Could you check a few things on this model? Use its own coordinates, in mm. Face numbers are marked on the shaded views. A direction names the side the tool comes from. Give positions to 0.01 mm unless a question says otherwise; leave off trailing zeros. Order: outer loops, then holes, each group sorted by start corner. A loop starts at its lowest first (then second) coordinate and runs counter-clockwise, first axis right, second up. Notation, with made-up numbers: (84, -30) -> (111, -30) arc R25 cw to (111, -13) -> close; hole circle Ø9 at (32.25, 10.5). An arc over 180 degrees is marked (long way). Write each question's results on one line, items separated by ' | '.
Autodesk Inventor part; units mm, degrees
ref_plane "YZ Plane" through (0, 0, 0) normal (1, 0, 0) x (0, 1, 0)
ref_plane "XZ Plane" through (0, 0, 0) normal (0, 1, 0) x (-1, 0, 0)
ref_plane "XY Plane" through (0, 0, 0) normal (0, 0, 1) x (1, 0, 0)
sketch "Schizzo1" plane through (0, 0, 0) normal (0, 1, 0) x (-1, 0, 0)
  line L0 (30.1714, 73.6571) -> (4.1714, 73.6571)
  line L1 (4.1714, 73.6571) -> (4.1714, -12.3429)
  line L2 (4.1714, -12.3429) -> (30.1714, -12.3429)
  line L3 (30.1714, -12.3429) -> (30.1714, 73.6571)
  line L4 (30.1714, 73.6571) -> (4.1714, -12.3429) construction
  line L5 (4.1714, 73.6571) -> (30.1714, -12.3429) construction
  point P0 (0, 0)
  point P1 (17.1714, 30.6571)
  dimension "d0" = 26
  dimension "d1" = 86
extrude "Estrusione1" add sketch "Schizzo1" along normal blind 20
sketch "Schizzo2" plane through (0, 0, 0) normal (0, -1, 0) x (1, 0, 0)
  line L0 (-4.1714, -12.3429) -> (-30.1714, -12.3429)
  line L1 (-4.1714, -12.3429) -> (-30.1714, -12.3429)
  line L2 (-30.1714, -12.3429) -> (-30.1714, 12.6571)
  line L3 (-30.1714, 12.6571) -> (-4.1714, 12.6571)
  line L4 (-4.1714, 12.6571) -> (-4.1714, -12.3429)
  line L5 (-30.1714, 73.6571) -> (-4.1714, 73.6571)
  line L6 (-4.1714, 73.6571) -> (-30.1714, 73.6571)
  line L7 (-30.1714, 73.6571) -> (-30.1714, 48.6571)
  line L8 (-30.1714, 48.6571) -> (-4.1714, 48.6571)
  line L9 (-4.1714, 48.6571) -> (-4.1714, 73.6571)
  point P0 (0, 0)
  dimension "d4" = 25
  dimension "d5" = 25
extrude "Estrusione2" add sketch "Schizzo2" along normal blind 25
sketch "Schizzo3" plane through (-30.1714, 20, 73.6571) normal (0, 0, 1) x (1, 0, 0)
  line L0 (0, -20) -> (0, -45)
  line L1 (0, -45) -> (26, -45)
  line L2 (0, -45) -> (26, -45)
  line L3 (26, -20) -> (26, -45)
  line L4 (26, -45) -> (26, -20)
  line L5 (26, -20) -> (0, -45)
  point P0 (30.1714, -20)
extrude "Estrusione3" cut sketch "Schizzo3" against normal through all
sketch "Schizzo4" plane through (-4.1714, 20, 73.6571) normal (1, 0, 0) x (0, 0, -1)
  line L0 (86, 0) -> (0, 0)
  line L1 (0, 0) -> (0, -10)
  line L2 (0, -45) -> (0, 0)
  line L3 (0, 0) -> (10, 0) construction
  line L4 (0, -10) -> (12, -10)
  line L5 (86, 0) -> (86, -10)
  line L6 (86, -45) -> (86, 0)
  line L7 (86, 0) -> (96, 0) construction
  line L8 (86, -10) -> (74, -10)
  circle A0 centre (12, -10) radius 2.5
  circle A1 centre (74, -10) radius 2.5
  point P0 (73.6571, -20)
  dimension "d10" = 10
  dimension "d11" = 90
  dimension "d12" = 12
  dimension "d13" = 90
  dimension "d14" = 10
  dimension "d15" = 90
  dimension "d16" = 12
  dimension "d17" = 90
  dimension "d18" = 5
  dimension "d19" = 5
hole "Foro1" at (-4.1714, 10, 61.6571) at (-4.1714, 10, -0.3429) direction (-1, 0, 0) diameter 5.9 end through all
sketch "Schizzo5" plane through (0, 20, 0) normal (0, 1, 0) x (1, 0, 0)
  line L0 (-30.1714, -73.6571) -> (-4.1714, -73.6571)
  line L1 (-30.1714, 12.3429) -> (-30.1714, -73.6571)
  line L2 (-30.1714, -73.6571) -> (-30.1714, 12.3429)
  line L3 (-30.1714, -30.6571) -> (-12.1714, -30.6571)
  line L4 (-30.1714, -30.6571) -> (-12.1714, -30.6571) construction
  point P0 (0, 0)
  dimension "d27" = 18
  dimension "d28" = 0
hole "Foro2" at (-12.1714, 20, 30.6571) direction (0, -1, 0) diameter 7 end through all
properties part number "23_Blocco_Escursione_Braccio_2"
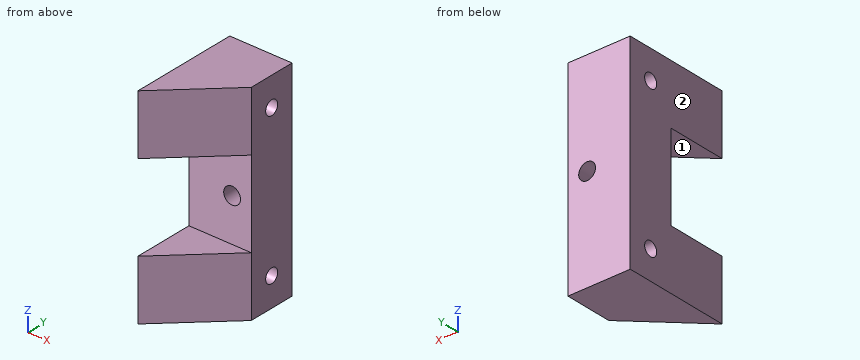
Q1. Suppose I cut it at C-C on x = -22. Please give me the cut outline in (y, z).
Here are the results:
outline: (-17.14, -12.34) -> (20, -12.34) -> (20, 73.66) -> (-17.14, 73.66) -> (-17.14, 48.66) -> (0, 48.66) -> (0, 12.66) -> (-17.14, 12.66) -> close; hole circle Ø5.9 at (10, -0.34); hole circle Ø5.9 at (10, 61.66)
Q2. For the marked faces 1 and 2, which set-ups out of +Z, -Z, +X, -X, +Y, -Y let a thin tool reach every point of the face, with its end or its side?
Here are the results:
face 1: +X, -X, -Y | face 2: +Z, -Z, -X, +Y, -Y
Q3. I need wall thicknesses on line 1 along Z through (x, y) = (-17.5, 10); line 2 along Z through (x, y) = (-9.25, 10); line 3 along Y through (x, z) = (-18.75, 35.5). Which ranges of each line are inside material? Lowest first, please.
Here are the results:
line 1: z = -12.34 to -3.29, 2.61 to 58.71, 64.61 to 73.66 | line 2: z = -12.34 to -3.29, 2.61 to 28.73, 32.58 to 58.71, 64.61 to 73.66 | line 3: y = 0 to 20
Q4. I'm going to push flat-ended pins straight in: pin 1 Ø8 at (x, z) = (-22.5, 39) entering from -Y; pin 2 Ø3 at (y, z) = (-13, 11) entering from +X; pin 3 Ø12 at (x, z) = (-13.5, 60.5) entering from -Y. Where does each tip first touch, or does it pass through?
Here are the results:
pin 1: stops at y = 0 | pin 2: stops at x = -16.13 | pin 3: stops at y = -14.74
Q5. Suppose I cut it at A-A on z = 32.5. Please give me the cut outline in (x, y).
Here are the results:
outline: (-30.17, 0) -> (-15.15, 0) -> (-15.15, 20) -> (-30.17, 20) -> close; (-9.2, 0) -> (-4.17, 0) -> (-4.17, 20) -> (-9.2, 20) -> close
Q6. Suppose I cut it at D-D on y = -6.5. Please give me the cut outline in (x, z), and give its area (3 significant figures).
Here are the results:
outline: (-30.17, -12.34) -> (-10.93, -12.34) -> (-10.93, 12.66) -> (-30.17, 12.66) -> close; (-30.17, 48.66) -> (-10.93, 48.66) -> (-10.93, 73.66) -> (-30.17, 73.66) -> close | area: 962 mm²
Q7. Suppose I cut it at B-B on y = 11. Please give me the cut outline in (x, z), and give its area (3 significant figures).
Here are the results:
outline: (-30.17, -12.34) -> (-4.17, -12.34) -> (-4.17, -3.12) -> (-30.17, -3.12) -> close; (-30.17, 2.43) -> (-4.17, 2.43) -> (-4.17, 58.88) -> (-30.17, 58.88) -> close; (-30.17, 64.43) -> (-4.17, 64.43) -> (-4.17, 73.66) -> (-30.17, 73.66) -> close; hole circle Ø7 at (-12.17, 30.66) | area: 1,910 mm²
